Could you check a few things on this drawing? It's one solid part, dimensions in mm from its lowest x, y, z. A direction names the side the tool comes from. Give positions to 0.01 mm unless a question says otherwise; leave off trailing zeros. Write each loop counter-clockwise with the first axis right and the second up, starting at its lowest first coordinate (ties: lowest second). Pieces come first, ordered by that corner, then holes. Notation, with made-up numbers: M 80,57 L 103,57 A22 ccw 103,90 Z; hole C 46.5,46.25 d4. An arc over 180 degrees is marked long. Use CSV: the item, a comma, the result in double quotes. Start each with the question number.
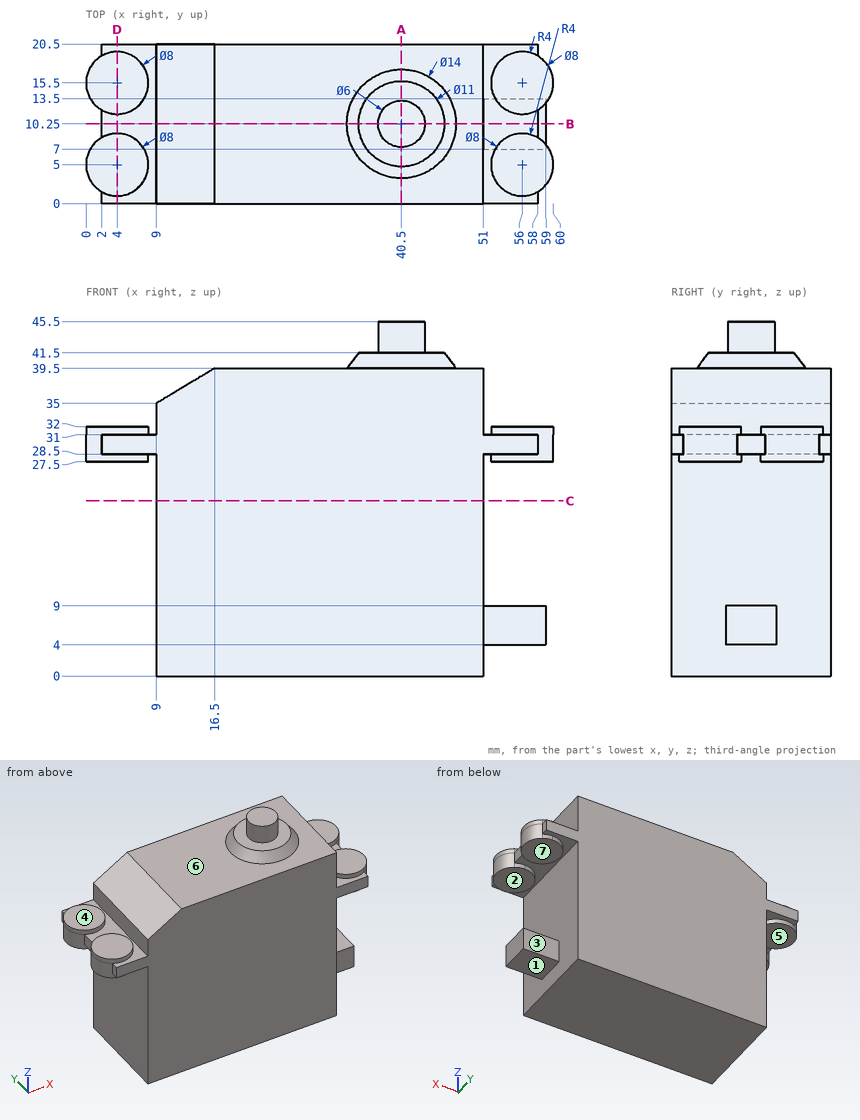
(1) I want a section at C-C (z = 22.5). Write out the boundary of the cut face in (x, y), and give its area (3 significant figures).
(2) I want a section at A-A (x = 40.5). Write out the boundary of the cut face in (y, z).
(3) Please list where these lines run through material, in increasing order: L1, parallel to X at y = 15.25, z = 18.5; L2, parallel to Z at x = 48, y = 16; L3, parallel to Z at x = 39, y = 13.75. Write a range as [from, to].
(4) I want a section at D-D (x = 4). Write out the boundary of the cut face in (y, z).
(5) Thinking about a two-plate mould opening in Z: for the marked faces 1, 2 and 3, which applies, released by +Z, released by -Z, zero draft, split by the parting line, or undercut?
(6) Will these pins go through, and if not, where does the flat tip stop? pin 1 Ø10.5 at (x, y) = (27.5, 11) entering from +Z; pin 2 Ø1.7 at (y, z) = (19.5, 30) entering from +X; pin 3 Ø10 at (y, z) = (17.5, 6.5) entering from +X.
(7) I want a section at B-B (y = 10.25). Write out the boundary of the cut face in (x, z), and give its area (3 significant figures).
(8) Which directions (+Z, -Z, +X, -X, +Y, -Y) give clear straight access to the entire face, cutting with the end or side of a thin tool? Please do the marked faces 4, 5, 6 and 7.
Geometry results:
1,outline,"M 9,0 L 51,0 L 51,20.5 L 9,20.5 Z"
1,area,"861 mm2"
2,outline,"M 0,0 L 20.5,0 L 20.5,39.5 L 17.25,39.5 L 15.75,41.5 L 13.25,41.5 L 13.25,45.5 L 7.25,45.5 L 7.25,41.5 L 4.75,41.5 L 3.25,39.5 L 0,39.5 Z"
3,L1,"x = [9, 51]"
3,L2,"z = [0, 39.5]"
3,L3,"z = [0, 41.5]"
4,outline,"M 0,28.5 L 1,28.5 L 1,27.5 L 9,27.5 L 9,28.5 L 11.5,28.5 L 11.5,27.5 L 19.5,27.5 L 19.5,28.5 L 20.5,28.5 L 20.5,31 L 19.5,31 L 19.5,32 L 11.5,32 L 11.5,31 L 9,31 L 9,32 L 1,32 L 1,31 L 0,31 Z"
5,face 1,"released by -Z"
5,face 2,"undercut"
5,face 3,"zero draft"
6,pin 1,"stops at z = 39.5"
6,pin 2,"stops at x = 58.47"
6,pin 3,"stops at x = 59"
7,outline,"M 2,28.5 L 9,28.5 L 9,0 L 51,0 L 51,4 L 59,4 L 59,9 L 51,9 L 51,28.5 L 58,28.5 L 58,31 L 51,31 L 51,39.5 L 47.5,39.5 L 46,41.5 L 43.5,41.5 L 43.5,45.5 L 37.5,45.5 L 37.5,41.5 L 35,41.5 L 33.5,39.5 L 16.5,39.5 L 9,35 L 9,31 L 2,31 Z"
7,area,"1,770 mm2"
8,face 4,"+Z, -X, +Y, -Y"
8,face 5,"-Z, -X, +Y, -Y"
8,face 6,"+Z"
8,face 7,"+X, +Y, -Y"
